from build123d import *

# Parameters (mm, degrees)
F0_R            = 76.3894607231
F1_DEPTH        = 25.4
F2_DEPTH        = 25.4
F4_DEPTH        = 50.8
F4_COPIES_COUNT = 20
F5_R            = 6.35
F6_R            = 2.54


# Not quite as in the source:
# - a pattern or mirror of a feature is missing from the dataset's text; its kind, count and spacing are read off the source's solid


with BuildPart() as f1:
    # F0 (on Top) → F1 (new body)
    with BuildSketch(Plane.XY):
        Circle(F0_R)
    extrude(amount=F1_DEPTH)

    # F2 (add): a face of the model
    f2_faces = [f1.faces().sort_by_distance(p)[0] for p in [
        (0, 0, 25.4),
    ]]
    extrude(f2_faces, amount=F2_DEPTH)

    # F3 (on face) → F4 (cut)
    with BuildSketch(Plane.XY.offset(50.8)):
        with BuildLine():
            ThreePointArc((5.0502526328, 76.2223370011), (-0.0057278173, 76.3894605084), (-5.0616831482, 76.2215787902))
            Line((-5.0616831482, 76.2215787902), (0, 57.8660437425))
            Line((0, 57.8660437425), (5.0502526328, 76.2223370011))
        make_face()
    f4 = extrude(amount=-F4_DEPTH, mode=Mode.SUBTRACT)

    # F4_copies: F4 ×20 about axis
    f4_copies_axis = Axis((0, 0, 0), (0, 0, 1))
    for i in range(1, F4_COPIES_COUNT):
        add(f4.rotate(f4_copies_axis, i * 360 / F4_COPIES_COUNT), mode=Mode.SUBTRACT)

    # F5
    f5_edges = [f1.edges().sort_by_distance(p)[0] for p in [
        (-5.061683, 76.221579, 25.4),
        (5.050253, 76.222337, 25.4),
        (-18.750922, 74.052364, 25.4),
        (18.739816, 74.055175, 25.4),
        (28.357073, 70.931136, 25.4),
        (40.706932, 64.639735, 25.4),
        (48.888106, 58.696702, 25.4),
        (58.68937, 48.896908, 25.4),
        (64.63363, 40.716625, 25.4),
        (70.926883, 28.36771, 25.4),
        (74.052364, 18.750922, 25.4),
        (76.221579, 5.061683, 25.4),
        (76.222337, -5.050253, 25.4),
        (74.055175, -18.739816, 25.4),
        (70.931136, -28.357073, 25.4),
        (64.639735, -40.706932, 25.4),
        (58.696702, -48.888106, 25.4),
        (48.896908, -58.68937, 25.4),
        (40.716625, -64.63363, 25.4),
        (28.36771, -70.926883, 25.4),
        (18.750922, -74.052364, 25.4),
        (5.061683, -76.221579, 25.4),
        (-5.050253, -76.222337, 25.4),
        (-18.739816, -74.055175, 25.4),
        (-28.357073, -70.931136, 25.4),
        (-40.706932, -64.639735, 25.4),
        (-48.888106, -58.696702, 25.4),
        (-58.68937, -48.896908, 25.4),
        (-64.63363, -40.716625, 25.4),
        (-70.926883, -28.36771, 25.4),
        (-74.052364, -18.750922, 25.4),
        (-76.221579, -5.061683, 25.4),
        (-76.222337, 5.050253, 25.4),
        (-74.055175, 18.739816, 25.4),
        (-70.931136, 28.357073, 25.4),
        (-64.639735, 40.706932, 25.4),
        (-58.696702, 48.888106, 25.4),
        (-48.896908, 58.68937, 25.4),
        (-40.716625, 64.63363, 25.4),
        (-28.36771, 70.926883, 25.4),
    ]]
    fillet(f5_edges, radius=F5_R)

    # F6
    f6_edges = [f1.edges().sort_by_distance(p)[0] for p in [
        (0, 57.866044, 25.4),
        (-17.881591, 55.033878, 25.4),
        (17.881591, 55.033878, 25.4),
        (-34.012807, 46.814613, 25.4),
        (34.012807, 46.814613, 25.4),
        (-46.814613, 34.012807, 25.4),
        (46.814613, 34.012807, 25.4),
        (-55.033878, 17.881591, 25.4),
        (55.033878, 17.881591, 25.4),
        (-57.866044, 0, 25.4),
        (57.866044, 0, 25.4),
        (-55.033878, -17.881591, 25.4),
        (55.033878, -17.881591, 25.4),
        (-46.814613, -34.012807, 25.4),
        (46.814613, -34.012807, 25.4),
        (-34.012807, -46.814613, 25.4),
        (34.012807, -46.814613, 25.4),
        (-17.881591, -55.033878, 25.4),
        (17.881591, -55.033878, 25.4),
        (0, -57.866044, 25.4),
    ]]
    fillet(f6_edges, radius=F6_R)


solid = f1.part
Source: CAD feature listing. Evaluate the final solid. Frame: model axes, mm. A direction names the side the tool comes from. Round coordinates to 2 decimals unless told otherwise and drop trailing zeros. Loops run counter-clockwise (first coordinate to the right, second up) from the corner with the lowest first, then second, coordinate; pieces in that order, holes last. Notation, with made-up numbers: M -7,34 L 1,34 A15 ccw 1,48 Z; hole C 17.5,48.25 d9. An arc over 180 degrees is marked long. Return JSON: item names as keys, results as strings. Group by question number.
1. Section query A-A on y = 0.5. Output: boundary loops of the cut face in (x, z), and give its area (3 significant figures).
2. Section query B-B on y = -31. Output: boundary loops of the cut face in (x, z).
3. Material intervals for line 1 along Y through (x, z) = (-64, 30); line 2 along Y through (x, z) = (63.5, 15.5); line 3 along Y through (x, z) = (-66, 23), sorted ascending. Write a range as from..to.
4. Reachability of faces 4 (the face through (38.844, -64.025, 25.044)), 5 (the face through (42.93, 53.94, 25.76)), 6 (the face through (-53.94, 42.93, 25.76)), 7 (the face through (-18.4, -66.5, 25.8)), 8 (the face through (-24.16, -64.56, 25.76)) from +Z, -Z, +X, -X, +Y, -Y: full face, straight path, thin tool, end or side. Return the list, or none.
5. Mould query, pull axis X, two halves, no side actions, for faces 1 (the face through (-64.56, 24.16, 25.76)), 2 (the face through (64.61, 24.2, 25.76)), 3 (the face through (-38.11, 52.52, 25.04)). Classes: released by +X, released by -X, zero draft, split by the parting line, or undercut.
6. Pin query (flat end, axial travel): pin 1 (10 mm diameter, centred on y = -46.5, z = 11, fed in from -X); pin 2 (4 mm diameter, centred on x = -21, z = 15.5, fed in from -Y); pin 3 (6 mm diameter, centred on x = -4.5, z = 42, fed in from +Y). Return the tip coordinate at first contact, or that it passes through.
Checks:
{
 "1": {"outline": "M -64.94,0 L 64.94,0 L 64.94,50.8 L -64.94,50.8 Z", "area": "6,600 mm²"},
 "2": {"outline": "M -69.29,0 L 69.29,0 L 69.29,50.8 L -69.29,50.8 Z"},
 "3": {"line 1": "y = -38.85..-23.8, -18.3..18.3, 23.79..38.85", "line 2": "y = -39..-23.46, -18.37..18.38, 23.47..39.01", "line 3": "y = -37.68..-25.12, -18.38..-2.1, 2.1..18.38, 25.11..37.68"},
 "4": {"face 4": "+Z, -Z, +X", "face 5": "+Z, -Z, +Y", "face 6": "+Z, -Z, -X", "face 7": "+Z, -Z", "face 8": "+Z, -Z, -Y"},
 "5": {"face 1": "released by -X", "face 2": "released by +X", "face 3": "undercut"},
 "6": {"pin 1": "stops at x = -56.73", "pin 2": "stops at y = -62.8", "pin 3": "stops at y = 75.29"}
}
